Model file for the job. Use its own axes, mm. A direction names the side the tool comes from. Coordinates: 2 decimals unless noted, no trailing zeros. Order: outer loops, then holes, each group sorted by start corner. A loop starts at its lowest first (then second) coordinate and runs counter-clockwise, first axis right, second up. Notation, with made-up numbers: (-27, 76.5) -> (27, 76.5) arc R19 ccw to (27, 107.5) -> close; hole circle Ø6 at (80.5, 80.5). An arc over 180 degrees is marked (long way). Write item = value, one per line. Start each with the question number.
Q1. Flat gauge pin, fed straight in: pin 1 (10 mm diameter, centred on x = -1.5, z = 23, fed in from +Y). Where does the tip first touch, or does it go through?
Q2. Mould opens along X. For faces 1 (the face through (-39.5, 2, 0)), 2 (the face through (-1, 0, 0)), 3 (the face through (-1, 2, -31.5)) say: +X half, -X half, draft (parallel to the pull), parting line (faces both ways), or undercut.
Q3. Wall check: line 1 (X direction, y = 1.6, z = -11.5); line 2 (Z direction, x = -23.5, y = 3.2); line 3 (Y direction, x = -29.5, z = -5.5). Give the ranges that are in metal, low to high. Write a range as from..to.
Q4. 3-axis set-ups, long thin cutter, end or side, ignore diameter. For faces 4 (the face through (-38.5, 2, 0)), 5 (the face through (-1, 2, -32.5)), 6 (the face through (3.75, 1, 32)): which of +Z, -Z, +X, -X, +Y, -Y reach the whole face in a straight line?
Q5. Cut at C-C, the plane z = -19.5. List the corners of the cut face in (x, y), plus the area to 3 significant figures.
Q6. Cut at A-A, the plane x = -12. List the corners of the cut face in (y, z), plus the area to 3 significant figures.
Q7. Cut at B-B, the plane y = 1.95. List the corners of the cut face in (x, z), plus the area to 4 significant figures.
from build123d import *

# Parameters (mm, degrees)
ESQUISSE1_W             = 79
ESQUISSE1_H             = 65
BOSS_EXTRU_1_DEPTH      = 3.5
ESQUISSE2_W             = 77
ESQUISSE2_H             = 63
ENL_V_MAT_EXTRU_1_DEPTH = 2.5
ESQUISSE3_W             = 7.5
ESQUISSE3_H             = 7.5
ENL_V_MAT_EXTRU_2_DEPTH = 1.25
CONG_1_R                = 5


with BuildPart() as part:
    # Esquisse1 → Boss.-Extru.1 (new body)
    with BuildSketch(Plane(origin=(0, 0, 0), x_dir=(1, 0, 0), z_dir=(0, 1, 0))):
        Rectangle(ESQUISSE1_W, ESQUISSE1_H)
    extrude(amount=BOSS_EXTRU_1_DEPTH)

    # Esquisse2 → Enlèv. mat.-Extru.1 (cut)
    with BuildSketch(Plane(origin=(0, 3.5, 0), x_dir=(1, 0, 0), z_dir=(0, 1, 0))):
        Rectangle(ESQUISSE2_W, ESQUISSE2_H)
    extrude(amount=-ENL_V_MAT_EXTRU_1_DEPTH, mode=Mode.SUBTRACT)

    # Esquisse3 → Enlèv. mat.-Extru.2 (cut)
    with BuildSketch(Plane.XY.offset(32.5)):
        with Locations((0, 1.75)):
            Rectangle(ESQUISSE3_W, ESQUISSE3_H)
    extrude(amount=-ENL_V_MAT_EXTRU_2_DEPTH, mode=Mode.SUBTRACT)

    # Congé1
    # the kernel refuses this fillet: 5 mm, written as the material it takes off along each edge
    with BuildSketch(Plane(origin=(-3.75, 1, 31.25), x_dir=(0, -1, 0), z_dir=(1, 0, 0))) as cong_1_piece_1:
        with BuildLine():
            CenterArc((5, 3), CONG_1_R, 180, 36.869897646)
            Line((0, 3), (-0.1, 3))
            Line((-0.1, 3), (-0.1, 0))
            Line((-0.1, 0), (0, -0.1))
            ThreePointArc((0, -0.1), (0.5, -0.1), (0.92, -0.06))
            Line((0.92, -0.06), (1, 0))
        make_face()
    extrude(amount=7.5, mode=Mode.SUBTRACT)


solid = part.part
Here are the results:
q1.pin_1 = 1
q2.face_1 = -X half
q2.face_2 = draft
q2.face_3 = undercut
q3.line_1 = -39.5..-38.5, 38.5..39.5
q3.line_2 = -32.5..-31.5, 31.5..32.5
q3.line_3 = 0..1
q4.face_4 = +Y
q4.face_5 = -Z, +X, -X, +Y, -Y
q4.face_6 = +Z, +Y
q5.outline = (-39.5, 0) -> (39.5, 0) -> (39.5, 3.5) -> (38.5, 3.5) -> (38.5, 1) -> (-38.5, 1) -> (-38.5, 3.5) -> (-39.5, 3.5) -> close
q5.area = 84.0 mm²
q6.outline = (0, -32.5) -> (3.5, -32.5) -> (3.5, -31.5) -> (1, -31.5) -> (1, 31.5) -> (3.5, 31.5) -> (3.5, 32.5) -> (0, 32.5) -> close
q6.area = 70.0 mm²
q7.outline = (-39.5, -32.5) -> (39.5, -32.5) -> (39.5, 32.5) -> (3.75, 32.5) -> (3.75, 31.5) -> (38.5, 31.5) -> (38.5, -31.5) -> (-38.5, -31.5) -> (-38.5, 31.5) -> (-3.75, 31.5) -> (-3.75, 32.5) -> (-39.5, 32.5) -> close
q7.area = 276.5 mm²
